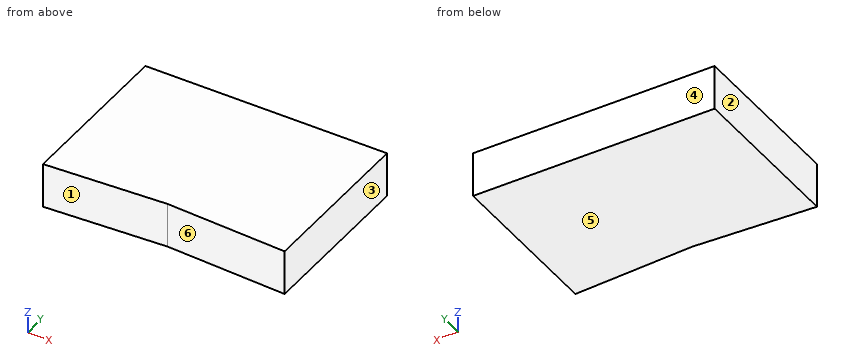
from build123d import *

# Parameters (mm, degrees)
SKETCH1_W           = 80
SKETCH1_H           = 14.88
BOSS_EXTRUDE1_DEPTH = 55.2
CUT_EXTRUDE1_DEPTH  = 70.774310459


with BuildPart() as part:
    # Sketch1 → Boss-Extrude1 (new body)
    with BuildSketch(Plane(origin=(0, 0, 0), x_dir=(1, 0, 0), z_dir=(0, 1, 0))):
        Rectangle(SKETCH1_W, SKETCH1_H)
    extrude(amount=-BOSS_EXTRUDE1_DEPTH)

    # Sketch3 → Cut-Extrude1 (cut, through all)
    with BuildSketch(Plane(origin=(0, 0, -7.44), x_dir=(-1, 0, 0), z_dir=(0, 0, -1))):
        Polygon((40, -55.2), (0, -53.103688829), (-40, -55.2), align=None)
    extrude(amount=-CUT_EXTRUDE1_DEPTH, mode=Mode.SUBTRACT)


solid = part.part
CAD build for the part. Positions are in the model's coordinates, mm. Face numbers are marked on the shaded views. A direction names the side the tool comes from. Give positions to 0.01 mm unless a question says otherwise; leave off trailing zeros. Write each loop counter-clockwise with the first axis right and the second up, starting at its lowest first coordinate (ties: lowest second). Pieces come first, ordered by that corner, then holes. Notation, with made-up numbers: (-36.75, -7) - (-12.75, -7) arc R5 ccw to (-12.75, -1) - close; hole circle Ø4 at (83, 28). An arc over 180 degrees is marked (long way). Answer as CSV lines item,"result".
Q1. Band-saw the part on C-C (x = -9). Give the cut face in (y, z).
Result set:
outline,"(-53.58, -7.44) - (0, -7.44) - (0, 7.44) - (-53.58, 7.44) - close"
Q2. Flat gauge pins, fed straight in: pin 1 Ø1 at (x, z) = (-22, 4.5) entering from +Y; pin 2 Ø6 at (x, z) = (-11.5, 4) entering from -Y; pin 3 Ø8 at (x, z) = (-13, 2.5) entering from -Y. Where does each tip first touch, or does it go through?
Result set:
pin 1,"y = 0"
pin 2,"y = -53.86"
pin 3,"y = -53.99"
Q3. 3-axis set-ups, long thin cutter, end or side, ignore diameter. For the marked faces 5 and 6: which of +Z, -Z, +X, -X, +Y, -Y reach the whole face in a straight line?
Result set:
face 5,"-Z, +X, -X, +Y, -Y"
face 6,"+Z, -Z, -Y"
Q4. Band-saw the part on B-B (x = 24). Give the cut face in (y, z).
Result set:
outline,"(-54.36, -7.44) - (0, -7.44) - (0, 7.44) - (-54.36, 7.44) - close"
Q5. Band-saw the part on A-A (z = 5.25). Give the cut face in (x, y).
Result set:
outline,"(-40, -55.2) - (0, -53.1) - (40, -55.2) - (40, 0) - (-40, 0) - close"
Q6. Drill centre lines: line 1 (Y direction, x = 11.5, z = 2.25); line 2 (Y direction, x = -36, z = -1.25). Where is each one in solid material? Low to high. Write a range as from..to.
Result set:
line 1,"-53.71..0"
line 2,"-54.99..0"
Q7. Pull direction X, two halves, no side cores. Call the marked faces 1, 2, 3 and 4: released by +X, released by -X, zero draft, split by the parting line, or undercut.
Result set:
face 1,"undercut"
face 2,"released by -X"
face 3,"released by +X"
face 4,"zero draft"
